```python
from build123d import *

# Parameters (mm, degrees)
F0_W      = 50
F0_H      = 100
F1_DEPTH  = 2
F2_W      = 2
F2_H      = 47
F3_DEPTH  = 28
F5_DEPTH  = 3
F7_DEPTH  = 3
F8_R      = 1.5
F9_DEPTH  = 60
F10_W     = 5
F10_H     = 5
F11_DEPTH = 12
F12_R     = 1
F13_DEPTH = 25
F14_R     = 1
F15_DEPTH = 25
F16_W     = 10
F16_H     = 15
F16_W_2   = 20
F16_H_2   = 20
F17_DEPTH = 25
F18_R     = 1.5
F18_W     = 10
F18_H     = 25
F19_DEPTH = 25
F20_W     = 3
F20_H     = 35
F21_DEPTH = 8
F22_R     = 2
F23_DEPTH = 100
F25_DEPTH = 3
F25_TAPER = -3
F27_DEPTH = 3
F28_R     = 2.45
F29_DEPTH = 3


with BuildPart() as f1:
    # F0 (on Top) → F1 (new body)
    with BuildSketch(Plane.XY):
        Polygon((25, 50), (25, -50), (50, -50), align=None)
        Polygon((-50, -50), (-25, -50), (-25, 50), align=None)
        Rectangle(F0_W, F0_H)
    extrude(amount=F1_DEPTH)

    # F2 (on Right) → F3 (join, symmetric)
    with BuildSketch(Plane.YZ):
        with Locations((-49, 23.5)):
            Rectangle(F2_W, F2_H)
    extrude(amount=F3_DEPTH, both=True)

    # F4 (on face) → F5 (join)
    with BuildSketch(Plane.YZ.offset(28)):
        with BuildLine():
            ThreePointArc((-48, 47.6458980338), (-49, 47.5), (-50, 47.6458980338))
            Line((-50, 47.6458980338), (-50, 47))
            Line((-50, 47), (-48, 47))
            Line((-48, 47), (-48, 47.6458980338))
        make_face()
        with BuildLine():
            ThreePointArc((-48, 47.6458980338), (-46.1937569599, 48.9083499337), (-45.5, 51))
            ThreePointArc((-45.5, 51), (-51.0916500663, 53.8062430401), (-50, 47.6458980338))
            ThreePointArc((-50, 47.6458980338), (-49, 47.5), (-48, 47.6458980338))
        make_face()
    extrude(amount=-F5_DEPTH)

    # F6 (on face) → F7 (join)
    with BuildSketch(Plane(origin=(-28, 0, 0), x_dir=(0, -1, 0), z_dir=(-1, 0, 0))):
        with BuildLine():
            ThreePointArc((50, 47.6458980338), (49, 47.5), (48, 47.6458980338))
            Line((48, 47.6458980338), (48, 47))
            Line((48, 47), (50, 47))
            Line((50, 47), (50, 47.6458980338))
        make_face()
        with BuildLine():
            ThreePointArc((50, 47.6458980338), (51.8062430401, 48.9083499337), (52.5, 51))
            ThreePointArc((52.5, 51), (46.9083499337, 53.8062430401), (48, 47.6458980338))
            ThreePointArc((48, 47.6458980338), (49, 47.5), (50, 47.6458980338))
        make_face()
    extrude(amount=-F7_DEPTH)

    # F8 (on face) → F9 (cut)
    with BuildSketch(Plane(origin=(-28, 0, 0), x_dir=(0, -1, 0), z_dir=(-1, 0, 0))):
        with Locations((49, 51)):
            Circle(F8_R)
    extrude(amount=-F9_DEPTH, mode=Mode.SUBTRACT)

    # F10 (on face) → F11 (join)
    with BuildSketch(Plane(origin=(0, -48, 0), x_dir=(-1, 0, 0), z_dir=(0, 1, 0))):
        with Locations((-5.5, 32.5)):
            Rectangle(F10_W, F10_H)
        with Locations((-5.5, 4.5)):
            Rectangle(F10_W, F10_H)
    extrude(amount=F11_DEPTH)

    # F12 (on face) → F13 (cut)
    with BuildSketch(Plane(origin=(3, 0, 0), x_dir=(0, -1, 0), z_dir=(-1, 0, 0))):
        with Locations((42, 4.5)):
            Circle(F12_R)
    extrude(amount=-F13_DEPTH, mode=Mode.SUBTRACT)

    # F14 (on face) → F15 (cut)
    with BuildSketch(Plane(origin=(3, 0, 0), x_dir=(0, -1, 0), z_dir=(-1, 0, 0))):
        with Locations((42, 32.5)):
            Circle(F14_R)
    extrude(amount=-F15_DEPTH, mode=Mode.SUBTRACT)

    # F16 (on face) → F17 (cut)
    with BuildSketch(Plane.XZ.offset(50)):
        with Locations((20, 39.5)):
            Rectangle(F16_W, F16_H)
        with Locations((-13, 14)):
            Rectangle(F16_W_2, F16_H_2)
    extrude(amount=-F17_DEPTH, mode=Mode.SUBTRACT)

    # F18 (on face) → F19 (cut)
    with BuildSketch(Plane.XY.offset(2)):
        with Locations((-20, -31)):
            Circle(F18_R)
        with Locations((-20, -6)):
            Circle(F18_R)
        with Locations((20, -31)):
            Circle(F18_R)
        with Locations((20, -6)):
            Circle(F18_R)
        with Locations((-31.5, -18.5)):
            Rectangle(F18_W, F18_H)
        with Locations((31.5, -18.5)):
            Rectangle(F18_W, F18_H)
    extrude(amount=-F19_DEPTH, mode=Mode.SUBTRACT)

    # F20 (on face) → F21 (join)
    with BuildSketch(Plane.XY.offset(2)):
        with Locations((-26, 16.5)):
            Rectangle(F20_W, F20_H)
        with Locations((0, 16.5)):
            Rectangle(F20_W, F20_H)
        with Locations((26, 16.5)):
            Rectangle(F20_W, F20_H)
    extrude(amount=F21_DEPTH)

    # F22 (on face) → F23 (cut)
    with BuildSketch(Plane(origin=(-27.5, 0, 0), x_dir=(0, -1, 0), z_dir=(-1, 0, 0))):
        with Locations((-29, 6)):
            Circle(F22_R)
        with Locations((-16.5, 6)):
            Circle(F22_R)
        with Locations((-4, 6)):
            Circle(F22_R)
    extrude(amount=-F23_DEPTH, mode=Mode.SUBTRACT)



with BuildPart() as f25:
    # F24 (on face) → F25 (new body)
    with BuildSketch(Plane.XZ.offset(50)):
        Polygon((48, 2), (28, 47.6458980338), (28, 2), align=None)
    extrude(amount=-F25_DEPTH, taper=F25_TAPER)


with BuildPart() as f25b:
    # F24 (on face) → F25, piece 2 (new body)
    with BuildSketch(Plane.XZ.offset(50)):
        Polygon((-28, 47.6458980338), (-48, 2), (-28, 2), align=None)
    extrude(amount=-F25_DEPTH, taper=F25_TAPER)


with BuildPart() as f1_1:
    add(f1.part)

    add(f25.part)  # F27 merges F25
    # F26 (on face) → F27 (join)
    with BuildSketch(Plane.YZ.offset(28)):
        with BuildLine():
            Line((-48, 2), (-32, 2))
            Line((-32, 2), (-45.6234731707, 51.9214480836))
            ThreePointArc((-45.6234731707, 51.9214480836), (-45.9408205628, 49.29958206), (-48, 47.6458980338))
            Line((-48, 47.6458980338), (-48, 2))
        make_face()
    extrude(amount=-F27_DEPTH)


    add(f25b.part)  # F29 merges F25b
    # F28 (on face) → F29 (join)
    with BuildSketch(Plane(origin=(-28, 0, 0), x_dir=(0, -1, 0), z_dir=(-1, 0, 0))):
        with BuildLine():
            Line((45.6234731707, 51.9214480836), (41.6528343038, 37.371557643))
            Line((41.6528343038, 37.371557643), (44.0563623479, 33.8951915058))
            ThreePointArc((44.0563623479, 33.8951915058), (44.3865148093, 33.2181203826), (44.5, 32.4734412134))
            ThreePointArc((44.5, 32.4734412134), (42.7353250903, 30.0840276846), (39.9325623907, 31.0678446383))
            Line((39.9325623907, 31.0678446383), (32, 2))
            Line((32, 2), (48, 2))
            Line((48, 2), (48, 47.6458980338))
            ThreePointArc((48, 47.6458980338), (45.9408205628, 49.29958206), (45.6234731707, 51.9214480836))
        make_face()
        with Locations((42, 4.5)):
            Circle(F28_R, mode=Mode.SUBTRACT)
    extrude(amount=-F29_DEPTH)


solid = f1_1.part
```
Build history of the part. All positions in model axes, mm. A direction names the side the tool comes from. Round coordinates to 2 decimals unless told otherwise and drop trailing zeros. Order: outer loops, then holes, each group sorted by start corner. A loop starts at its lowest first (then second) coordinate and runs counter-clockwise, first axis right, second up. Notation, with made-up numbers: (23.5, 36.5) - (28.5, 36.5) arc R24 cw to (28.5, 50.5) - close; hole circle Ø1 at (-9, -33). An arc over 180 degrees is marked (long way). Use a Markdown table: item, result.
1) Wall check: L1, parallel to X at y = 25, z = 6; L2, parallel to Z at x = -26.9, y = 4; L3, parallel to Z at x = 4.5, y = -42. Give the ranges that are in metal, low to high.
Recorded:
| item | result |
|---|---|
| L1 | x = -27.5 to -24.5, -1.5 to 1.5, 24.5 to 27.5 |
| L2 | z = 0 to 4, 8 to 10 |
| L3 | z = 0 to 3.5, 5.5 to 7, 30 to 31.5, 33.5 to 35 |
2) Saw through at B-B on x = -20. Write the cut outline in (y, z), and give its area (3 significant figures).
Recorded:
| item | result |
|---|---|
| outline | (-50, 0) - (-32.5, 0) - (-32.5, 2) - (-48, 2) - (-48, 4) - (-50, 4) - close; (-50, 24) - (-48, 24) - (-48, 47) - (-50, 47) - close; (-29.5, 0) - (-7.5, 0) - (-7.5, 2) - (-29.5, 2) - close; (-4.5, 0) - (50, 0) - (50, 2) - (-4.5, 2) - close |
| area | 238 mm² |
3) Pull direction Y, two halves, no side cores. Call faces 1 (the face through (24.5, 16, 3)), 2 (the face through (-26.521, -36.022, 16.737)), 3 (the face through (6, -36, 5)), 4 (the face through (26.5, -47.8, 50.1)): pulls with the +Y half, pulls with the -Y half, needs draft (parallel to the pull), parting line crosses it, or undercut.
Recorded:
| item | result |
|---|---|
| face 1 | needs draft |
| face 2 | undercut |
| face 3 | pulls with the +Y half |
| face 4 | undercut |
4) Saw through at A-A on y = 4. Write the cut outline in (x, z).
Recorded:
| item | result |
|---|---|
| outline | (-36.5, 0) - (36.5, 0) - (36.5, 2) - (27.5, 2) - (27.5, 4) - (24.5, 4) - (24.5, 2) - (1.5, 2) - (1.5, 4) - (-1.5, 4) - (-1.5, 2) - (-24.5, 2) - (-24.5, 4) - (-27.5, 4) - (-27.5, 2) - (-36.5, 2) - close; (-27.5, 8) - (-24.5, 8) - (-24.5, 10) - (-27.5, 10) - close; (-1.5, 8) - (1.5, 8) - (1.5, 10) - (-1.5, 10) - close; (24.5, 8) - (27.5, 8) - (27.5, 10) - (24.5, 10) - close |
5) Flat gauge pins, fed straight in: pin 1 Ø5 at (y, z) = (4, 6) entering from +X; pin 2 Ø0.9 at (x, z) = (0.5, 7.5) entering from +Y; pin 3 Ø1.5 at (x, y) = (-0.5, -17) entering from +Z; pin 4 Ø12 at (x, y) = (-4.5, 13.5) entering from -Z. Where does each tip first touch, or does it go through?
Recorded:
| item | result |
|---|---|
| pin 1 | stops at x = 27.5 |
| pin 2 | stops at y = 34 |
| pin 3 | stops at z = 2 |
| pin 4 | stops at z = 0 |
6) Saw through at C-C on y = 20. Write the cut outline in (x, z).
Recorded:
| item | result |
|---|---|
| outline | (-32.5, 0) - (32.5, 0) - (32.5, 2) - (27.5, 2) - (27.5, 10) - (24.5, 10) - (24.5, 2) - (1.5, 2) - (1.5, 10) - (-1.5, 10) - (-1.5, 2) - (-24.5, 2) - (-24.5, 10) - (-27.5, 10) - (-27.5, 2) - (-32.5, 2) - close |
7) Tool access for faces 5 (the face through (-27.5, 16, 3)), 6 (the face through (27.5, 16, 3)), 7 (the face through (26, 17, 10)), 8 (the face through (6, -42, 7)), 9 (the face through (8, -42, 31)): list every direction of +Z, -Z, +X, -X, +Y, -Y with a clear straight run to the whole face (end or side of a thin tool).
Recorded:
| item | result |
|---|---|
| face 5 | +Z, -X, +Y |
| face 6 | +Z, +X, +Y |
| face 7 | +Z, +X, -X, +Y |
| face 8 | +Y |
| face 9 | +Z, +Y |
